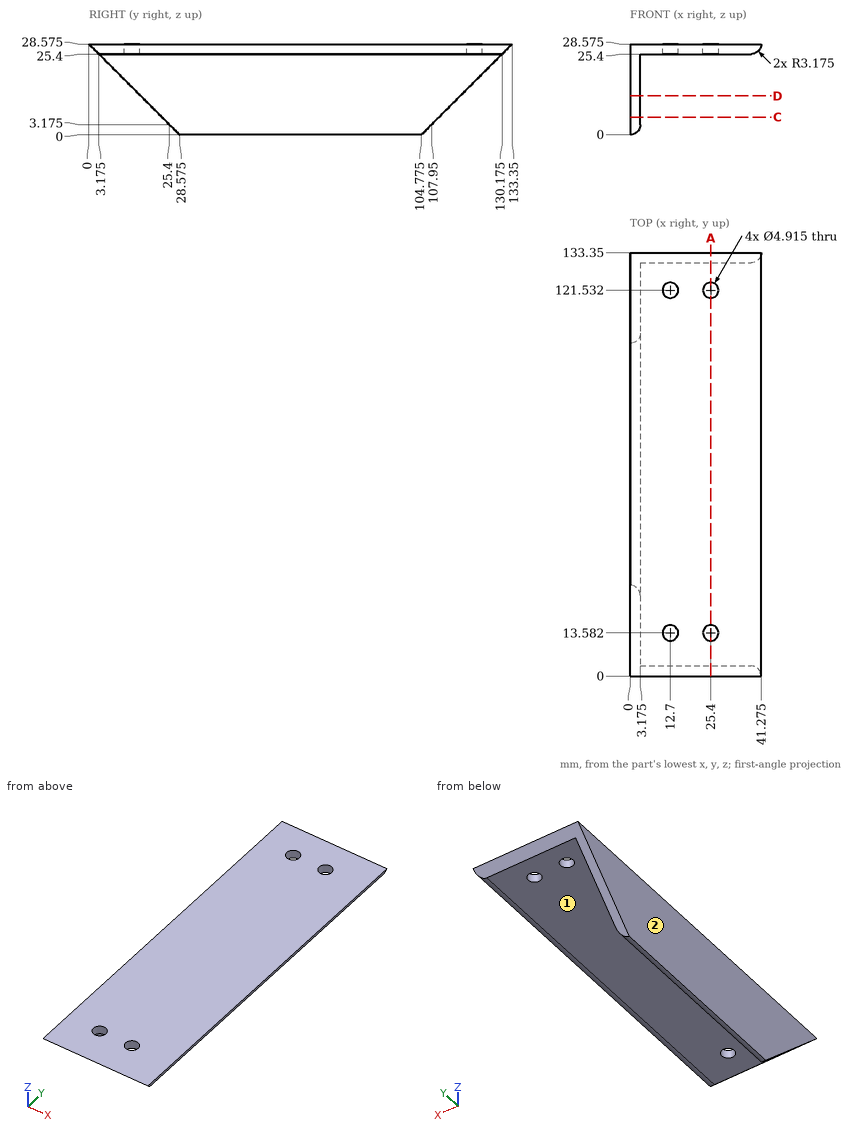
Geometry: see drawing. Coordinates: mm, zero at the bounding-box minimum. A direction names the side the tool comes from. Give positions to 0.01 mm unless a question says otherwise; leave off trailing zeros. Order: outer loops, then holes, each group sorted by start corner. A loop starts at its lowest first (then second) coordinate and runs counter-clockwise, first axis right, second up. Notation, with made-up numbers: (52.5, 48.5) -> (72.5, 48.5) arc R26 cw to (72.5, 73.5) -> close; hole circle Ø10 at (-15.75, 57). An arc over 180 degrees is marked (long way). Write each question's results on one line, items separated by ' | '. Start each with the question number.
1) First-contact query: pin 1 (6 mm diameter, centred on y = 119, z = 12.5, fed in from +X) (3 decimals); pin 2 (6.5 mm diameter, centred on x = 12.7, y = 13.58, fed in from -Z). Flat tips, straight axial feed; report the tip coordinate or a pass-through.
2) Section C-C (z = 5.5). Return loops of the section in (x, y) (3 decimals), then the cut area to 3 significant figures.
3) Section D-D (z = 12.25). Return loops of the section in (x, y) (3 decimals), then the cut area to 3 significant figures.
4) Line query: line 1 (Y direction, x = 25.4, z = 27.45) (1 decimal); line 2 (Z direction, x = 6, y = 19) (3 decimals); line 3 (Y direction, x = 12.7, z = 27.8) (1 decimal). Output: solid intervals per line, ascending. Write a range as from..to.
5) Section A-A (x = 25.4). Count the separate pieces of the cut face and the enclosed holes in it, then the cut area to 3 significant figures.
6) Set-up query: the marked faces 1 and 2. Return all of +Z, -Z, +X, -X, +Y, -Y with unobstructed straight access to the full face (end or side cutting, diameter ignored); none if empty.
Calculated:
1) pin 1: x = 3.175 | pin 2: z = 25.4
2) outline: (0, 23.075) -> (3.175, 23.075) -> (3.175, 110.275) -> (0, 110.275) -> close | area: 277 mm2
3) outline: (0, 16.325) -> (3.175, 16.325) -> (3.175, 117.025) -> (0, 117.025) -> close | area: 320 mm2
4) line 1: 1.1..11.1, 16..119.1, 124..132.2 | line 2: 25.4..28.575 | line 3: 0.8..11.1, 16..119.1, 124..132.6
5) separate pieces: 3 | enclosed holes: 0 | area: 382 mm2
6) face 1: -Z, +X, +Y, -Y | face 2: +Z, -Z, -X, +Y, -Y
